Job drawing, mm, ordinate dimensions from the low corner. One solid piece. A direction names the side the tool comes from. Round coordinates to 2 decimals unless told otherwise and drop trailing zeros. Order: outer loops, then holes, each group sorted by start corner. A loop starts at its lowest first (then second) coordinate and runs counter-clockwise, first axis right, second up. Notation, with made-up numbers: (7.25, 4) -> (54.25, 4) arc R24 cw to (54.25, 40) -> close; hole circle Ø11 at (-12.75, 54.25). An arc over 180 degrees is marked (long way). Write item = value, one per line.
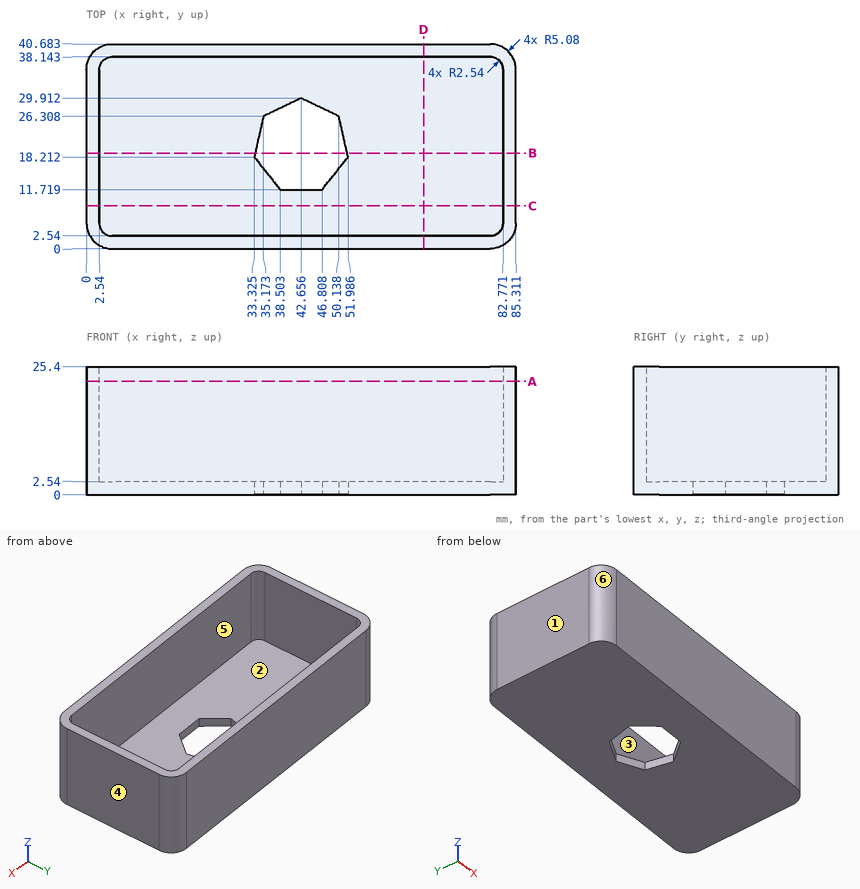
Q1. Cut at A-A, the plane z = 22.5. List the corners of the cut face in (x, y).
Check values:
outline = (0, 5.08) arc R5.08 ccw to (5.08, 0) -> (80.23, 0) arc R5.08 ccw to (85.31, 5.08) -> (85.31, 35.6) arc R5.08 ccw to (80.23, 40.68) -> (5.08, 40.68) arc R5.08 ccw to (0, 35.6) -> close; hole (2.54, 5.08) arc R2.54 ccw to (5.08, 2.54) -> (80.23, 2.54) arc R2.54 ccw to (82.77, 5.08) -> (82.77, 35.6) arc R2.54 ccw to (80.23, 38.14) -> (5.08, 38.14) arc R2.54 ccw to (2.54, 35.6) -> close
Q2. Flat gauge pin, fed straight in: pin 1 (10.5 mm diameter, centred on x = 61.5, y = 29, fed in from +Z). Where does the tip first touch, or does it go through?
Check values:
pin_1 = 2.54
Q3. Which spindle directions (+Z, -Z, +X, -X, +Y, -Y) get a long thin tool onto all of the face, cutting with end or side? Do the marked faces 5 and 6. Say none if no direction does.
Check values:
face_5 = +Z
face_6 = +Z, -Z, -X, -Y
Q4. Probe probe 1 along X at (y, z) = (29.5, 9); probe 2 along Y at (x, z) = (16.5, 3.75); probe 3 along Z at (x, y) = (72, 36). List the from-to ranges inside material, lowest first.
Check values:
probe_1 = 0 to 2.54, 82.77 to 85.31
probe_2 = 0 to 2.54, 38.14 to 40.68
probe_3 = 0 to 2.54
Q5. Cut at C-C, the plane y = 8.5. List the corners of the cut face in (x, z).
Check values:
outline = (0, 0) -> (85.31, 0) -> (85.31, 25.4) -> (82.77, 25.4) -> (82.77, 2.54) -> (2.54, 2.54) -> (2.54, 25.4) -> (0, 25.4) -> close
Q6. Cut at B-B, the plane y = 19. List the corners of the cut face in (x, z) (1 decimal).
Check values:
outline = (0, 0) -> (33.5, 0) -> (33.5, 2.5) -> (2.5, 2.5) -> (2.5, 25.4) -> (0, 25.4) -> close; (51.8, 0) -> (85.3, 0) -> (85.3, 25.4) -> (82.8, 25.4) -> (82.8, 2.5) -> (51.8, 2.5) -> close
Q7. Cut at D-D, the plane x = 67. List the corners of the cut face in (y, z).
Check values:
outline = (0, 0) -> (40.68, 0) -> (40.68, 25.4) -> (38.14, 25.4) -> (38.14, 2.54) -> (2.54, 2.54) -> (2.54, 25.4) -> (0, 25.4) -> close
Q8. Mould opens along X. For the marked faces 1, 2, 3 and 4 say: released by +X, released by -X, zero draft, split by the parting line, or undercut.
Check values:
face_1 = released by -X
face_2 = undercut
face_3 = undercut
face_4 = released by +X
